Here's how the part is built. I have some questions about the finished solid (model axes, mm). Face numbers are marked on the shaded views. A direction names the side the tool comes from. Give positions to 0.01 mm unless a question says otherwise; leave off trailing zeros. Write each loop counter-clockwise with the first axis right and the second up, starting at its lowest first coordinate (ties: lowest second). Pieces come first, ordered by that corner, then holes. Notation, with made-up numbers: (14.5, 46.25) -> (59.5, 46.25) arc R26 cw to (59.5, 60.25) -> close; hole circle Ø5 at (66.25, -23). An arc over 180 degrees is marked (long way). Put each result on its own line as item: value. Start each with the question number.
from build123d import *

# Parameters (mm, degrees)
F1_DEPTH = 50
F5_R     = 5


# Not quite as in the source:
# - the program builds the solid bodies; features that only make, move or delete a surface that nothing else refers to are left out


with BuildPart() as f1:
    # F0 (on Top) → F1 (new body)
    with BuildSketch(Plane.XY):
        with BuildLine():
            ThreePointArc((9.9498743711, 49), (0, 40), (-9.9498743711, 49))
            ThreePointArc((-9.9498743711, 49), (-35.3553390593, 35.3553390593), (-49, 9.9498743711))
            ThreePointArc((-49, 9.9498743711), (-40, 0), (-49, -9.9498743711))
            ThreePointArc((-49, -9.9498743711), (-35.3553390593, -35.3553390593), (-9.9498743711, -49))
            ThreePointArc((-9.9498743711, -49), (0, -40), (9.9498743711, -49))
            ThreePointArc((9.9498743711, -49), (35.3553390593, -35.3553390593), (49, -9.9498743711))
            ThreePointArc((49, -9.9498743711), (40, 0), (49, 9.9498743711))
            ThreePointArc((49, 9.9498743711), (35.3553390593, 35.3553390593), (9.9498743711, 49))
        make_face()
        with BuildLine():
            ThreePointArc((-4.9607837082, -19.375), (-14.1421356237, -14.1421356237), (-19.375, -4.9607837082))
            ThreePointArc((-19.375, -4.9607837082), (-25, 0), (-19.375, 4.9607837082))
            ThreePointArc((-19.375, 4.9607837082), (-14.1421356237, 14.1421356237), (-4.9607837082, 19.375))
            ThreePointArc((-4.9607837082, 19.375), (0, 25), (4.9607837082, 19.375))
            ThreePointArc((4.9607837082, 19.375), (14.1421356237, 14.1421356237), (19.375, 4.9607837082))
            ThreePointArc((19.375, 4.9607837082), (25, 0), (19.375, -4.9607837082))
            ThreePointArc((19.375, -4.9607837082), (14.1421356237, -14.1421356237), (4.9607837082, -19.375))
            ThreePointArc((4.9607837082, -19.375), (0, -25), (-4.9607837082, -19.375))
        make_face(mode=Mode.SUBTRACT)
    extrude(amount=F1_DEPTH)

    # F5
    f5_edges = [f1.edges().sort_by_distance(p)[0] for p in [
        (35.355339, -35.355339, 50),
        (35.355339, 35.355339, 50),
        (-35.355339, -35.355339, 50),
        (-35.355339, 35.355339, 50),
    ]]
    fillet(f5_edges, radius=F5_R)


solid = f1.part
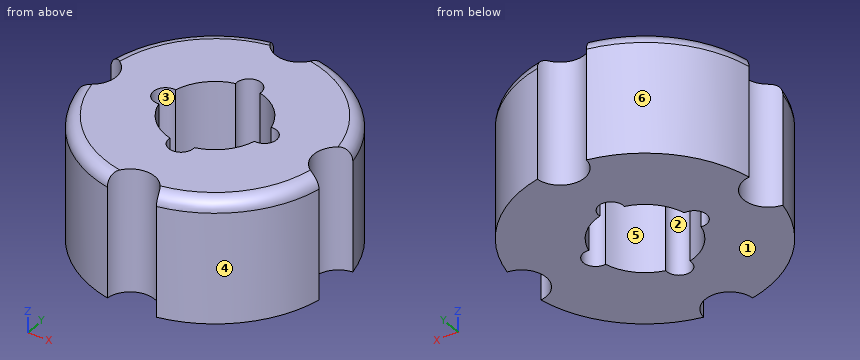
1) I'm going to push flat-ended pins straight in: pin 1 Ø8 at (x, y) = (0, 20) entering from +Z; pin 2 Ø12 at (y, z) = (25, 22) entering from -X; pin 3 Ø1.5 at (x, z) = (-19, 30) entering from -Y; pin 4 Ø2 at (x, z) = (25, 39) entering from +Y. Where does each tip first touch, or does it pass through?
2) I want a section at A-A, the plane y = 0. Write out the boundary of the cut face in (x, z).
3) I want a section at C-C, the plane z = 28.5. Write out the boundary of the cut face in (x, y) (3 decimals).
4) Thinking about a two-plate mould opening in Y: for the marked faces 1, 2, 3 and 4, which applies, released by +Y, released by -Y, zero draft, split by the parting line, or undercut?
5) Which directions (+Z, -Z, +X, -X, +Y, -Y) give clear straight access to the entire face, cutting with the end or side of a thin tool? Please do the marked faces 5 and 6.
6) I need wall thicknesses on probe 1 along Y at (x, z) = (-12, 36); probe 2 along Y at (x, z) = (-24.5, 16.5); probe 3 along X at (y, z) = (16.5, 25.5). Which ranges of each line are inside material? Lowest first, please.
Established:
1. pin 1: passes through
1. pin 2: stops at x = -46.25
1. pin 3: stops at y = -46.55
1. pin 4: stops at y = 43.86
2. outline: (-40, 0) -> (-25, 0) -> (-25, 50) -> (-40, 50) -> close; (25, 0) -> (40, 0) -> (40, 50) -> (25, 50) -> close
3. outline: (-49, -9.95) arc R50 ccw to (-9.95, -49) arc R10 cw to (9.95, -49) arc R50 ccw to (49, -9.95) arc R10 cw to (49, 9.95) arc R50 ccw to (9.95, 49) arc R10 cw to (-9.95, 49) arc R50 ccw to (-49, 9.95) arc R10 cw to start; hole (-19.375, -4.961) arc R20 ccw to (-4.961, -19.375) arc R5 ccw (long way) to (4.961, -19.375) arc R20 ccw to (19.375, -4.961) arc R5 ccw (long way) to (19.375, 4.961) arc R20 ccw to (4.961, 19.375) arc R5 ccw (long way) to (-4.961, 19.375) arc R20 ccw to (-19.375, 4.961) arc R5 ccw (long way) to start
4. face 1: zero draft
4. face 2: undercut
4. face 3: undercut
4. face 4: released by -Y
5. face 5: +Z, -Z
5. face 6: +Z, -Z, -X, +Y
6. probe 1: y = -48.54 to -16, 16 to 48.54
6. probe 2: y = -43.59 to -2.18, 2.18 to 43.59
6. probe 3: x = -47.2 to -11.3, 11.3 to 47.2
